Print and shaded views of the part. All mm, measured from the part's lowest x, y and z. Round coordinates to 2 decimals unless told otherwise and drop trailing zeros. Write each loop counter-clockwise with the first axis right and the second up, starting at its lowest first coordinate (ties: lowest second). Pieces come first, ordered by that corner, then holes. Notation, with made-up numbers: M -18.5,72 L 30.5,72 A26 cw 30.5,111 Z; hole C -4,-5 d9. An arc over 180 degrees is marked long. Write item = value, one per line.
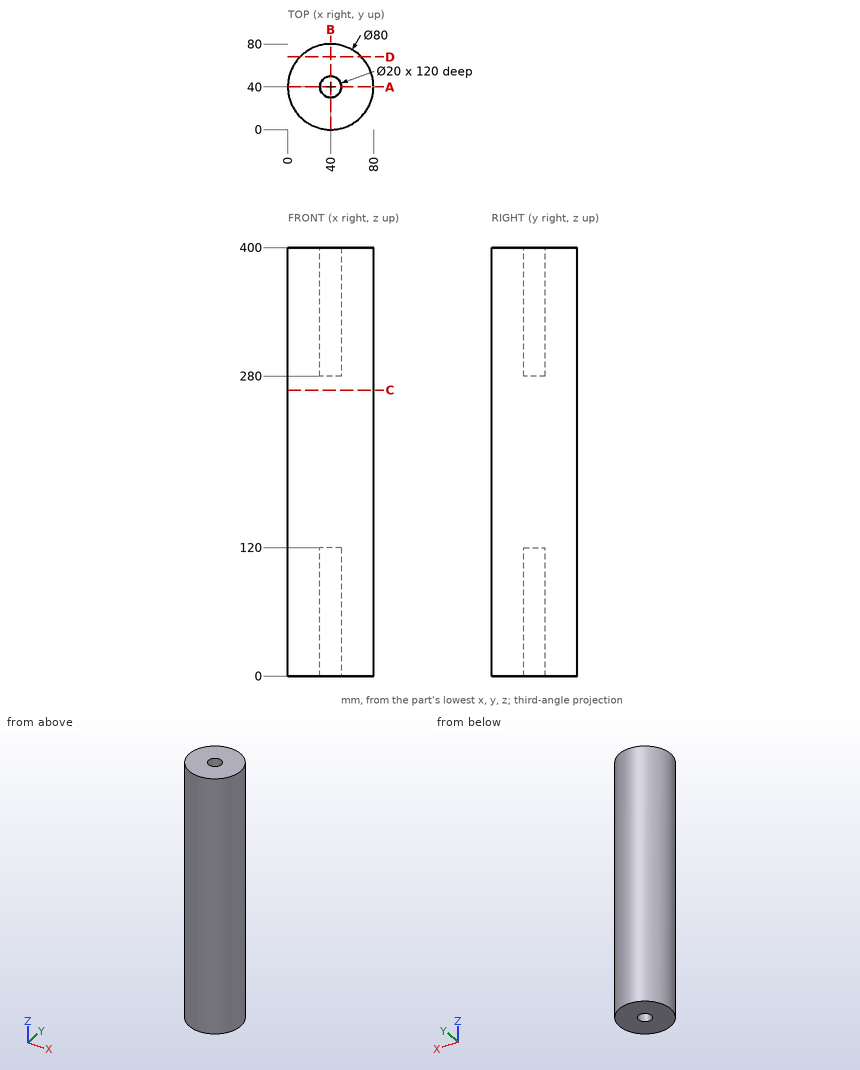
1. Probe probe 1 along Y at (x, z) = (40.5, 326.5); probe 2 along Y at (x, z) = (44.5, 91); probe 3 along X at (y, z) = (37, 340). List the from-to ranges inside material, lowest first.
Responses:
probe_1 = 0 to 30.01, 49.99 to 80
probe_2 = 0.25 to 31.07, 48.93 to 79.75
probe_3 = 0.11 to 30.46, 49.54 to 79.89
2. Band-saw the part on D-D (y = 68). List the corners of the cut face in (x, z), plus the area to 3 significant figures.
Responses:
outline = M 11.43,0 L 68.57,0 L 68.57,400 L 11.43,400 Z
area = 22,900 mm²
3. Band-saw the part on A-A (y = 40). List the corners of the cut face in (x, z).
Responses:
outline = M 0,0 L 30,0 L 30,120 L 50,120 L 50,0 L 80,0 L 80,400 L 50,400 L 50,280 L 30,280 L 30,400 L 0,400 Z
4. Band-saw the part on C-C (z = 267). List the corners of the cut face in (x, y).
Responses:
outline = C 40,40 d80
5. Flat gauge pins, fed straight in: pin 1 (1 mm diameter, centred on y = 59, z = 45.5, fed in from -X); pin 2 (10 mm diameter, centred on x = 42, z = 181, fed in from +Y); pin 3 (6 mm diameter, centred on y = 20, z = 233.5, fed in from -X). Where does each tip first touch, or does it go through?
Responses:
pin_1 = 4.54
pin_2 = 80
pin_3 = 3.79
